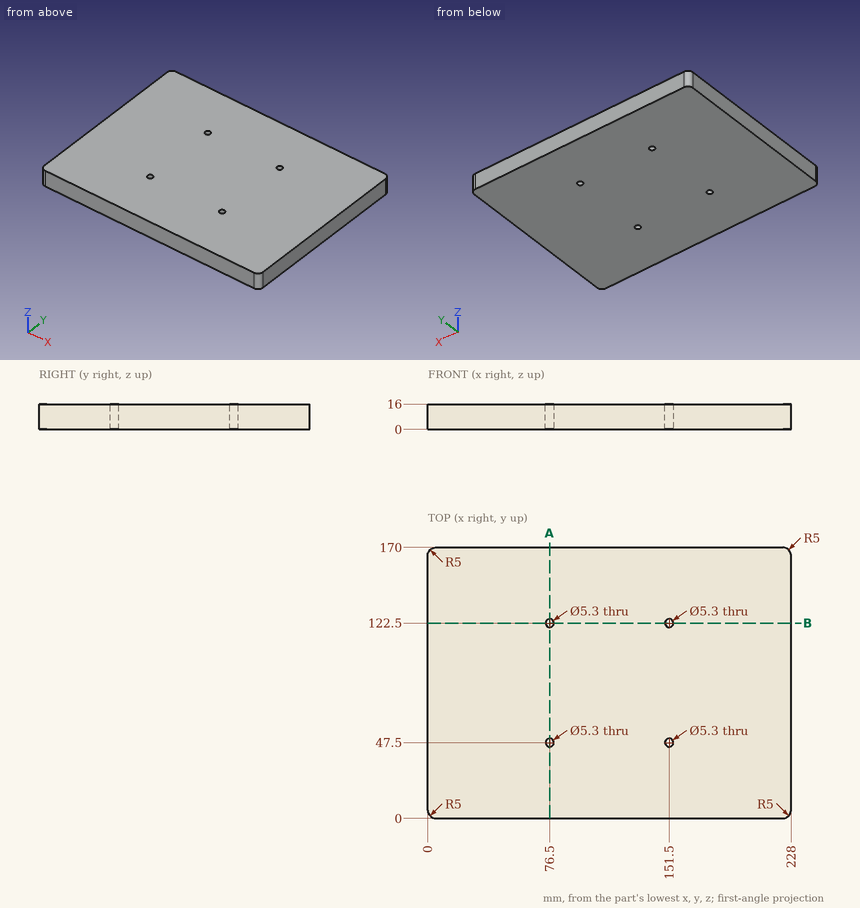
Source: three-view drawing plus pictorial views. Frame: mm from the lowest corner of the part. Round coordinates to 2 decimals unless told otherwise and drop trailing zeros. Loops run counter-clockwise (first coordinate to the right, second up) from the corner with the lowest first, then second, coordinate; pieces in that order, holes last.
1. Section query B-B on y = 122.5. Output: boundary loops of the cut face in (x, z), and give its area (3 significant figures).
2. Section query A-A on x = 76.5. Output: boundary loops of the cut face in (y, z), and give its area (3 significant figures).
3. Ray query, L1, parallel to Y at x = 151.5, z = 10.25. Return the intervals inside material, ascending.
Answers below:
1. outline: (0, 0) - (73.85, 0) - (73.85, 16) - (0, 16) - close; (79.15, 0) - (148.85, 0) - (148.85, 16) - (79.15, 16) - close; (154.15, 0) - (228, 0) - (228, 16) - (154.15, 16) - close
1. area: 3,480 mm2
2. outline: (0, 0) - (44.85, 0) - (44.85, 16) - (0, 16) - close; (50.15, 0) - (119.85, 0) - (119.85, 16) - (50.15, 16) - close; (125.15, 0) - (170, 0) - (170, 16) - (125.15, 16) - close
2. area: 2,550 mm2
3. L1: y = 0 to 44.85, 50.15 to 119.85, 125.15 to 170
